Design review of the part built by this model. Coordinates are the model's own, in mm. A direction names the side the tool comes from. Round coordinates to 2 decimals unless told otherwise and drop trailing zeros. Write each loop counter-clockwise with the first axis right and the second up, starting at its lowest first coordinate (ties: lowest second). Pieces come first, ordered by that corner, then holes. Notation, with made-up numbers: (8, 67) - (63, 67) arc R15 cw to (63, 96) - close; hole circle Ø6 at (30.25, -38). An arc over 180 degrees is marked (long way). Use one line per item in the form item = value.
```python
from build123d import *

# Parameters (mm, degrees)
EXTRUDE_1_DEPTH            = 90
HOLE_WIZARD_M52_AT_2_COUNT = 2
HOLE_WIZARD_M52_AT_2_PITCH = 63
HOLE_WIZARD_M52_AT_3_COUNT = 2
HOLE_WIZARD_M52_AT_3_PITCH = 93
HOLE_WIZARD_M52_AT_4_COUNT = 2
HOLE_WIZARD_M52_AT_4_PITCH = 156


with BuildPart() as part:
    # Эскиз1 → Бобышка-Вытянуть1 (new body, symmetric)
    with BuildSketch(Plane.XY):
        Polygon((4, 0), (-4, 0), (-4, -2.8), (-9.65, -2.8), (-9.65, -4.3), (-4, -9.3), (4, -9.3), (9.65, -4.3), (9.65, -2.8), (4, -2.8), align=None)
    extrude(amount=EXTRUDE_1_DEPTH, both=True)

    # Эскиз6 → Отверстие обработанное метчиком M52 (revolve, cut)
    with BuildSketch(Plane(origin=(0, 0, -78), x_dir=(0, 0, 1), z_dir=(1, 0, 0))):
        Polygon((0, 0), (0, 9.3), (2.525, 9.3), (2.1, 8.875), (2.1, 0.425), (2.525, 0), align=None)
    hole_wizard_m52 = revolve(axis=Axis((0, 6.35, -78), (0, -1, 0)), mode=Mode.SUBTRACT)

    # Отверстие обработанное метчиком M52 at 2: Отверстие обработанное метчиком M52 ×2
    with Locations(*[(0, 0, i * HOLE_WIZARD_M52_AT_2_PITCH) for i in range(1, HOLE_WIZARD_M52_AT_2_COUNT)]):
        add(hole_wizard_m52, mode=Mode.SUBTRACT)

    # Отверстие обработанное метчиком M52 at 3: Отверстие обработанное метчиком M52 ×2
    with Locations(*[(0, 0, i * HOLE_WIZARD_M52_AT_3_PITCH) for i in range(1, HOLE_WIZARD_M52_AT_3_COUNT)]):
        add(hole_wizard_m52, mode=Mode.SUBTRACT)

    # Отверстие обработанное метчиком M52 at 4: Отверстие обработанное метчиком M52 ×2
    with Locations(*[(0, 0, i * HOLE_WIZARD_M52_AT_4_PITCH) for i in range(1, HOLE_WIZARD_M52_AT_4_COUNT)]):
        add(hole_wizard_m52, mode=Mode.SUBTRACT)


solid = part.part
```
Q1. We need section A-A on z = 78. Write out the cut boundary in (x, y) (3 decimals).
Calculated:
outline = (-9.65, -4.3) - (-4, -9.3) - (-2.525, -9.3) - (-2.1, -8.875) - (-2.1, -0.425) - (-2.525, 0) - (-4, 0) - (-4, -2.8) - (-9.65, -2.8) - close; (2.1, -8.875) - (2.525, -9.3) - (4, -9.3) - (9.65, -4.3) - (9.65, -2.8) - (4, -2.8) - (4, 0) - (2.525, 0) - (2.1, -0.425) - close
Q2. We need section C-C on z = -63. Write out the cut boundary in (x, y).
Calculated:
outline = (-9.65, -4.3) - (-4, -9.3) - (4, -9.3) - (9.65, -4.3) - (9.65, -2.8) - (4, -2.8) - (4, 0) - (-4, 0) - (-4, -2.8) - (-9.65, -2.8) - close
Q3. We need section B-B on y = -6. Write out the cut boundary in (x, z), then the cut area to 3 significant figures.
Calculated:
outline = (-7.73, -90) - (7.73, -90) - (7.73, 90) - (-7.73, 90) - close; hole circle Ø4.2 at (0, -78); hole circle Ø4.2 at (0, -15); hole circle Ø4.2 at (0, 15); hole circle Ø4.2 at (0, 78)
area = 2,730 mm2
Q4. We need section D-D on x = 0. State how many separate pieces and enclosed holes the cut face has, then the cut area to 3 significant figures.
Calculated:
separate_pieces = 5
enclosed_holes = 0
area = 1,520 mm2
Q5. Draft analysis for pull direction Z (two halves, no side actions). For faces 1 (the cylindrical face through (-0.09, -4.59, 75.9)), 2 (the flat face through (0, -5, -90)), 3 (the flat face through (4, -1, 1)), state which applies: released by +Z, released by -Z, zero draft, split by the parting line, or undercut.
Calculated:
face_1 = undercut
face_2 = released by -Z
face_3 = zero draft
Q6. For P1, Ø2, axis at x = 7, z = 63.5, coming from the -Y side; P2, Ø6, axis at x = 8, z = -28.5, coming from the +Y side; P3, Ø0.8, axis at y = -2, z = 12.5, coming from the -X side, all flat-tipped, find the tip position at first contact; note any pin that passes through.
Calculated:
P1 = -7.53
P2 = -2.8
P3 = -4
Q7. To check wall thickness, follow line 1 along Z through (x, y) = (-0.25, -2); line 2 along X through (y, z) = (-4.25, 15); line 3 along X through (y, z) = (-5.75, 15). State the ranges of each line that lie inside material, in increasing order. Write a range as from..to.
Calculated:
line_1 = -90..-80.09, -75.91..-17.09, -12.91..12.91, 17.09..75.91, 80.09..90
line_2 = -9.65..-2.1, 2.1..9.65
line_3 = -8.01..-2.1, 2.1..8.01
Q8. Machinability: for faces 4 (the flat face through (7, -2.8, 1)), 5 (the flat face through (-7, -2.8, 1)), 6 (the cylindrical face through (-0.09, -4.59, 12.9)), which of the approach directions +Z, -Z, +X, -X, +Y, -Y give a long, thin tool a straight path to every point of the face, cutting with its end or side? Answer none if there is none.
Calculated:
face_4 = +Z, -Z, +X, +Y
face_5 = +Z, -Z, -X, +Y
face_6 = +Y, -Y
